Autodesk Inventor part; units mm, degrees
ref_plane "Arbeitsebene1" through (9.5, 0, 0) normal (1, 0, 0) x (0, 1, 0)
ref_plane "Arbeitsebene2" through (0, 9.5, 0) normal (0, 1, 0) x (-1, 0, 0)
ref_plane "XY Plane" through (0, 0, 0) normal (0, 0, 1) x (1, 0, 0)
sketch "Skizze1" plane through (0, 0, 0) normal (0, 1, 0) x (-1, 0, 0)
  line L0 (0, 0) -> (8, 0)
  line L1 (8, 0) -> (8, -59)
  line L2 (8, -59) -> (9.5, -59)
  line L3 (9.5, -59) -> (9.5, -293)
  line L4 (9.5, -293) -> (8, -293)
  line L5 (8, -293) -> (8, -352)
  line L6 (8, -352) -> (0, -352)
  line L7 (0, -352) -> (0, 0)
  dimension "d0" = 16
  dimension "d1" = 59
  dimension "d2" = 59
  dimension "d3" = 352
  dimension "d4" = 19
revolve "Umdrehung1" add sketch "Skizze1" angle 360 about axis through (0, 0, -352) along (0, 0, 1)
ref_plane "Arbeitsebene1" through (9.5, 0, 0) normal (1, 0, 0) x (0, 1, 0)
sketch "Skizze2" plane through (9.5, 0, 0) normal (1, 0, 0) x (0, 1, 0)
  line L0 (8, 0) -> (-8, 0)
  point P0 (0, 0)
  point P1 (0, -69)
  point P2 (0, 0)
  dimension "d7" = 69
hole "Bohrung1" at (9.5, 0, -69) direction (-1, 0, 0) diameter 8 end through all
ref_plane "Arbeitsebene2" through (0, 9.5, 0) normal (0, 1, 0) x (-1, 0, 0)
sketch "Skizze3" plane through (0, 9.5, 0) normal (0, 1, 0) x (-1, 0, 0)
  line L0 (9.5, -293) -> (-9.5, -293)
  point P0 (0, 0)
  point P1 (0, -283)
  dimension "d16" = 10
hole "Bohrung2" at (0, 9.5, -283) direction (0, -1, 0) diameter 8 end through all
properties part number "2011"
Read the model definition and answer for the solid it produces. Units are mm, in the model's axes. A direction names the side the tool comes from. Round coordinates to 2 decimals unless told otherwise and drop trailing zeros. Order: outer loops, then holes, each group sorted by start corner. A loop starts at its lowest first (then second) coordinate and runs counter-clockwise, first axis right, second up. Notation, with made-up numbers: (12, -25.5) - (23, -25.5) arc R18 ccw to (23, -7.5) - close; hole circle Ø10 at (-32, -18). An arc over 180 degrees is marked (long way). Use one line per item in the form item = value. Start each with the question number.
(1) The part is cut by section C-C (z = -35). Give the vertices of the cut face in (x, y).
(2) The part is cut by section D-D (z = -270). Give the vertices of the cut face in (x, y).
(3) For faces 1 (the face through (4.3, 7, -293)), 2 (the face through (4.3, 7, -59)), 3 (the face through (0, 0, -287)), determine the directions among +Z, -Z, +X, -X, +Y, -Y from which every point of the face is accessible in a straight line to the end or side of a thin tool.
(4) The part is cut by section B-B (y = 0). Give the vertices of the cut face in (x, z), then the cut area to 3 significant figures.
(5) Flat-ended cylindrical pins translate along their axes: pin 1 Ø1 at (x, z) = (2.5, -212.5) entering from -Y; pin 2 Ø5 at (x, z) = (5, -206) entering from +Y; pin 3 Ø1.5 at (x, z) = (-3.5, -74.5) entering from -Y. Find the tip coordinate at first contact, or state that the pin passes through.
(6) The part is cut by section A-A (x = 0). Give the vertices of the cut face in (y, z), then the cut area to 3 significant figures.
(7) Determine the mould class of faces 4 (the face through (1.73, -7.81, -29.91)), 5 (the face through (0, 0, 0)), 6 (the face through (-0.133, 1.532, -72.695)) for opening direction Y: +Y half, -Y half, draft (parallel to the pull), parting line (faces both ways), or undercut.
(8) Find the intervals of material crossed by line 1 along Z through (x, y) = (-4.25, 0); line 2 along Y through (x, z) = (0.5, -69); line 3 along Z through (x, y) = (0, 1), in increasing order. Write a range as from..to.
Checked values:
q1.outline = circle Ø16 at (0, 0)
q2.outline = circle Ø19 at (0, 0)
q3.face_1 = -Z
q3.face_2 = +Z
q3.face_3 = +Y, -Y
q4.outline = (-9.5, -293) - (-8, -293) - (-8, -352) - (8, -352) - (8, -293) - (9.5, -293) - (9.5, -73) - (-9.5, -73) - close; (-9.5, -65) - (9.5, -65) - (9.5, -59) - (8, -59) - (8, 0) - (-8, 0) - (-8, -59) - (-9.5, -59) - close; hole circle Ø8 at (0, -283)
q4.area = 6,130 mm^2
q5.pin_1 = -9.29
q5.pin_2 = 9.17
q5.pin_3 = -9.09
q6.outline = (-9.5, -293) - (-8, -293) - (-8, -352) - (8, -352) - (8, -293) - (9.5, -293) - (9.5, -287) - (-9.5, -287) - close; (-9.5, -279) - (9.5, -279) - (9.5, -59) - (8, -59) - (8, 0) - (-8, 0) - (-8, -59) - (-9.5, -59) - close; hole circle Ø8 at (0, -69)
q6.area = 6,130 mm^2
q7.face_4 = parting line
q7.face_5 = draft
q7.face_6 = undercut
q8.line_1 = -352..-73, -65..0
q8.line_2 = -9.49..-4, 4..9.49
q8.line_3 = -352..-287, -279..-72.87, -65.13..0
